```python
from build123d import *

# Parameters (mm, degrees)
F1_DEPTH = 47.625
F2_R     = 3.4925
F3_DEPTH = 25.4
F4_R     = 3.4925
F5_DEPTH = 25.4


with BuildPart() as f1:
    # F0 (on Top) → F1 (new body)
    with BuildSketch(Plane.XY):
        Polygon((38.1, 0), (0, 0), (0, -3.175), (0, -38.1), (3.175, -38.1), (3.175, -3.175), (38.1, -3.175), align=None)
    extrude(amount=F1_DEPTH)

    # F2 (on face) → F3 (cut)
    with BuildSketch(Plane(origin=(0, 0, 0), x_dir=(-1, 0, 0), z_dir=(0, 1, 0))):
        with Locations((-12.7, 42.8625)):
            Circle(F2_R)
        with Locations((-25.4, 23.8125)):
            Circle(F2_R)
        with Locations((-12.7, 4.7625)):
            Circle(F2_R)
    extrude(amount=-F3_DEPTH, mode=Mode.SUBTRACT)

    # F4 (on face) → F5 (cut)
    with BuildSketch(Plane(origin=(0, 0, 0), x_dir=(0, -1, 0), z_dir=(-1, 0, 0))):
        with Locations((12.7, 42.8625)):
            Circle(F4_R)
        with Locations((25.4, 23.8125)):
            Circle(F4_R)
        with Locations((12.7, 4.7625)):
            Circle(F4_R)
    extrude(amount=-F5_DEPTH, mode=Mode.SUBTRACT)


solid = f1.part
```
Geometry: final body of the model. Coordinates: model frame, mm. A direction names the side the tool comes from. Give positions to 0.01 mm unless a question says otherwise; leave off trailing zeros. Loops run counter-clockwise (first coordinate to the right, second up) from the corner with the lowest first, then second, coordinate; pieces in that order, holes last. Notation, with made-up numbers: (34.5, 87.5) - (73.5, 87.5) arc R11 cw to (73.5, 102.5) - close; hole circle Ø3 at (26, 9). An arc over 180 degrees is marked (long way). Answer as CSV lines item,"result". Start each with the question number.
(1) Section query A-A (y = -12.7). Output: boundary loops of the cut face in (x, z) (3 decimals).
(2) Mould query, pull axis Z, two halves, no side actions, for faces 3 (the face through (1.565, -12.245, 46.325)), 4 (the face through (20, -3.175, 23)), 5 (the face through (2, -10, 0)), 6 (the face through (1.565, -10.126, 7.123)). Classes: +Z half, -Z half, draft (parallel to the pull), parting line (faces both ways), or undercut.
(3) Reachability of faces 1 (the face through (28.89, -1.57, 23.97)), 2 (the face through (3.175, -21, 23)) from +Z, -Z, +X, -X, +Y, -Y: full face, straight path, thin tool, end or side. Return the list, or none.
(4) Section query D-D (z = 23). Output: boundary loops of the cut face in (x, y) (3 decimals).
(5) Pin query (flat end, axial travel): P1, Ø1.5, axis at x = 25, z = 15.5, coming from the -Y side (3 decimals); P2, Ø4, axis at x = 25.4, z = 23.81, coming from the +Y side; P3, Ø10, axis at y = -27.5, z = 23, coming from the +X side (3 decimals). Return the tip coordinate at first contact, or that it passes through.
(6) Section query B-B (x = 12.7). Output: boundary loops of the cut face in (y, z) (3 decimals), and give its area (3 significant figures).
(7) Ray query, line 1 along Z through (x, y) = (1.9, -12.7) (3 decimals); line 2 along Z through (x, y) = (1, -12) (3 decimals); line 3 along Y through (x, z) = (21, 33.5) (3 decimals). Return the intervals inside material, ascending. Write a range as [from, to].
(8) Section query C-C (x = 25.4). Output: boundary loops of the cut face in (y, z) (3 decimals), and give its area (3 significant figures).
Worked answers:
1,outline,"(0, 0) - (3.175, 0) - (3.175, 1.27) - (0, 1.27) - close; (0, 8.255) - (3.175, 8.255) - (3.175, 39.37) - (0, 39.37) - close; (0, 46.355) - (3.175, 46.355) - (3.175, 47.625) - (0, 47.625) - close"
2,face 3,"undercut"
2,face 4,"draft"
2,face 5,"-Z half"
2,face 6,"undercut"
3,face 1,"+Y, -Y"
3,face 2,"+Z, -Z, +X, -Y"
4,outline,"(0, -38.1) - (3.175, -38.1) - (3.175, -28.797) - (0, -28.797) - close; (0, -22.003) - (3.175, -22.003) - (3.175, -3.175) - (22.003, -3.175) - (22.003, 0) - (0, 0) - close; (28.797, -3.175) - (38.1, -3.175) - (38.1, 0) - (28.797, 0) - close"
5,P1,"stops at y = -3.175"
5,P2,"passes through"
5,P3,"stops at x = 3.175"
6,outline,"(-3.175, 0) - (0, 0) - (0, 1.27) - (-3.175, 1.27) - close; (-3.175, 8.255) - (0, 8.255) - (0, 39.37) - (-3.175, 39.37) - close; (-3.175, 46.355) - (0, 46.355) - (0, 47.625) - (-3.175, 47.625) - close"
6,area,"107 mm^2"
7,line 1,"z = [0, 1.27], [8.255, 39.37], [46.355, 47.625]"
7,line 2,"z = [0, 1.341], [8.184, 39.441], [46.284, 47.625]"
7,line 3,"y = [-3.175, 0]"
8,outline,"(-3.175, 0) - (0, 0) - (0, 20.32) - (-3.175, 20.32) - close; (-3.175, 27.305) - (0, 27.305) - (0, 47.625) - (-3.175, 47.625) - close"
8,area,"129 mm^2"
